The drawing under review shows one solid part. Ordinate dimensions are in mm from its lowest x, y, z. A direction names the side the tool comes from. Round coordinates to 2 decimals unless told otherwise and drop trailing zeros. Order: outer loops, then holes, each group sorted by start corner. A loop starts at its lowest first (then second) coordinate and runs counter-clockwise, first axis right, second up.
1) To check wall thickness, follow L1, parallel to X at y = 3, z = 2.78; L2, parallel to Z at x = 3.65, y = 4.75; L3, parallel to Y at x = 3.45, z = 4.9. State the ranges of each line that lie inside material, in increasing order.
2) Clearance check with a flat-ended pin moving along its axis: P1, Ø1, axis at y = 2.5, z = 1, coming from the -X side. State where the tip first meets the part, or that it passes through.
3) Machinability: for the marked faces 1 and 2, which of the approach directions +Z, -Z, +X, -X, +Y, -Y give a long, thin tool a straight path to every point of the face, cutting with its end or side? Answer none if there is none.
4) Consider section A-A (x = 2.78). Give the boundary of the cut face in (y, z) (3 decimals).
5) Consider section C-C (y = 3). Give the boundary of the cut face in (x, z), then the cut area to 3 significant figures.
6) Consider section B-B (z = 2.78). Give the boundary of the cut face in (x, y) (3 decimals), then the cut area to 3 significant figures.
7) Consider section D-D (x = 4.45). Give the boundary of the cut face in (y, z).
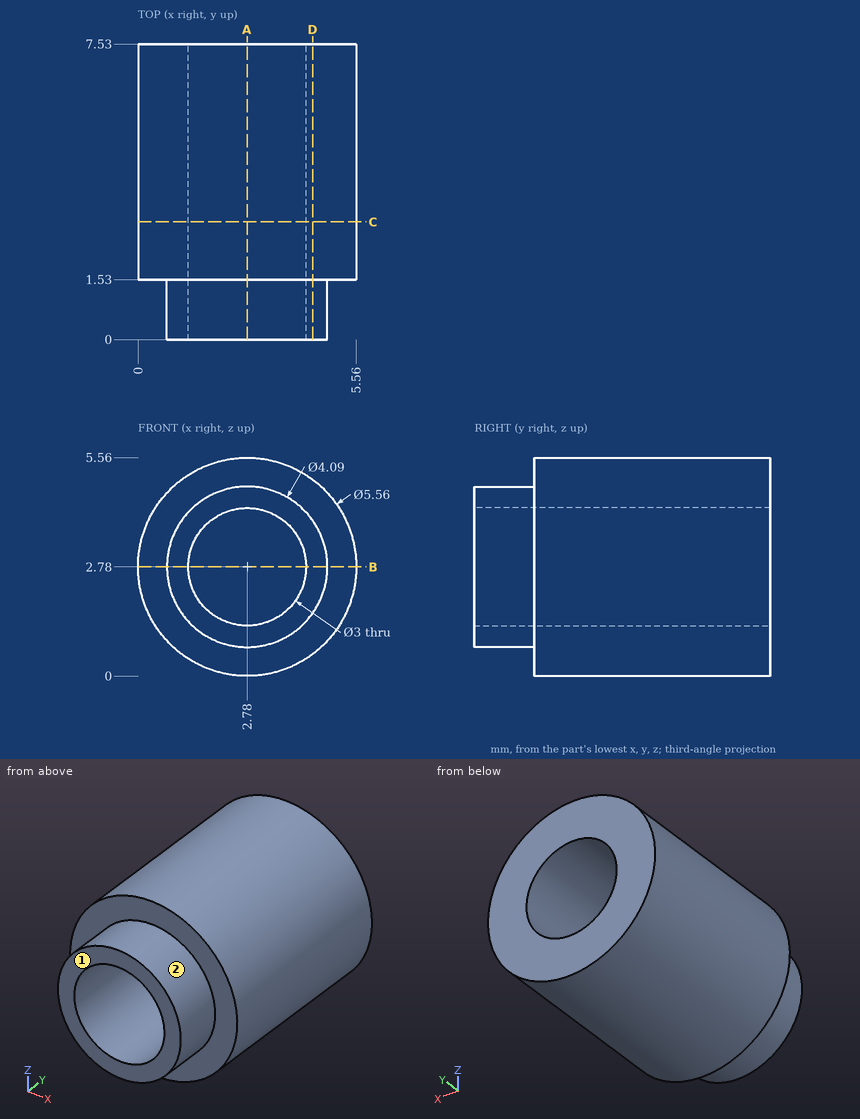
Answer below:
1. L1: x = 0 to 1.28, 4.28 to 5.56
1. L2: z = 0.14 to 1.56, 4 to 5.42
1. L3: y = 1.53 to 7.53
2. P1: stops at x = 0.31
3. face 1: +Z, -Z, +X, -X, -Y
3. face 2: -Y
4. outline: (0, 0.735) - (1.53, 0.735) - (1.53, 0) - (7.53, 0) - (7.53, 1.28) - (0, 1.28) - close; (0, 4.28) - (7.53, 4.28) - (7.53, 5.56) - (1.53, 5.56) - (1.53, 4.825) - (0, 4.825) - close
5. outline: circle Ø5.56 at (2.78, 2.78); hole circle Ø3 at (2.78, 2.78)
5. area: 17.2 mm2
6. outline: (0, 1.53) - (0.735, 1.53) - (0.735, 0) - (1.28, 0) - (1.28, 7.53) - (0, 7.53) - close; (4.28, 0) - (4.825, 0) - (4.825, 1.53) - (5.56, 1.53) - (5.56, 7.53) - (4.28, 7.53) - close
6. area: 17.0 mm2
7. outline: (0, 1.6) - (1.53, 1.6) - (1.53, 0.56) - (7.53, 0.56) - (7.53, 5) - (1.53, 5) - (1.53, 3.96) - (0, 3.96) - close
